Read the model definition and answer for the solid it produces. Units are mm, in the model's axes. A direction names the side the tool comes from. Round coordinates to 2 decimals unless told otherwise and drop trailing zeros. Write each loop counter-clockwise with the first axis right and the second up, starting at its lowest first coordinate (ties: lowest second). Pieces come first, ordered by that corner, then holes. Notation, with made-up numbers: (-1.75, 77.25) -> (43.25, 77.25) arc R4 ccw to (43.25, 82.25) -> close; hole circle Ø3 at (-38, 18). An arc over 180 degrees is marked (long way). Return JSON: item names as keys, results as strings.
from build123d import *

# Parameters (mm, degrees)
F0_R     = 6.3627
F1_DEPTH = 8.9916
F2_R     = 5.08
F3_DEPTH = 33.02
F4_DEPTH = 33.02


with BuildPart() as f1:
    # F0 (on Top) → F1 (new body)
    with BuildSketch(Plane.XY):
        Circle(F0_R)
    extrude(amount=-F1_DEPTH)

    # F2 (on Right) → F3 (join)
    with BuildSketch(Plane.YZ):
        with Locations((0, -3.8867404219)):
            Circle(F2_R)
    extrude(amount=F3_DEPTH)

    # F4 (cut, through all): a face of the model
    f4_faces = [f1.faces().sort_by_distance(p)[0] for p in [
        (0, 0, 0.4824606672),
    ]]
    extrude(f4_faces, amount=-F4_DEPTH, mode=Mode.SUBTRACT)


solid = f1.part
Item 1: Flat-ended cylindrical pins translate along their axes: pin 1 (1.5 mm diameter, centred on x = 6.5, y = 3.5, fed in from +Z); pin 2 (3 mm diameter, centred on x = 15, y = -4.5, fed in from -Z). Find the tip coordinate at first contact, or state that the pin passes through.
Worked answers:
{"pin 1": "stops at z = 0", "pin 2": "stops at z = -7.99"}
Item 2: Straight lines are drawn through the part: L1, parallel to Z at x = 19, y = -0.25; L2, parallel to Y at x = 29, z = -3.5; L3, parallel to Y at x = 8, z = -0.5. For each, find the intervals that lie inside material, in ascending order. Write a range as [from, to].
Worked answers:
{"L1": "z = [-8.96, 0]", "L2": "y = [-5.07, 5.07]", "L3": "y = [-3.79, 3.79]"}
Item 3: Section D-D (y = 2.5) is taken. Give the vertices of the cut face in (x, z), then the cut area to 3 significant figures.
Worked answers:
{"outline": "(-5.85, -8.99) -> (5.85, -8.99) -> (5.85, -8.31) -> (33.02, -8.31) -> (33.02, 0) -> (-5.85, 0) -> close", "area": "331 mm2"}
Item 4: A tool of negligible diameter and unlimited length cuts with its end or side. For faces 1 (the flat face through (13, 0, 0)), 2 (the cylindrical face through (18.221, -0.174, -8.964)), from which of +Z, -Z, +X, -X, +Y, -Y can it reach the whole face along a straight path? Write none if from no direction.
Worked answers:
{"face 1": "+Z, +X, -X, +Y, -Y", "face 2": "+X"}
Item 5: Section B-B (z = -3) is taken. Give the vertices of the cut face in (x, y), then the cut area to 3 significant figures.
Worked answers:
{"outline": "(3.93, -5) -> (33.02, -5) -> (33.02, 5) -> (3.93, 5) arc R6.36 ccw (long way) to start", "area": "401 mm2"}
Item 6: Section C-C (x = 11) is taken. Give the vertices of the cut face in (y, z), then the cut area to 3 significant figures.
Worked answers:
{"outline": "(-3.27, 0) arc R5.08 ccw (long way) to (3.27, 0) -> close", "area": "75.7 mm2"}
Item 7: Section A-A (y = 4.5) is taken. Give the vertices of the cut face in (x, z).
Worked answers:
{"outline": "(-4.5, -8.99) -> (4.5, -8.99) -> (4.5, -6.24) -> (33.02, -6.24) -> (33.02, -1.53) -> (4.5, -1.53) -> (4.5, 0) -> (-4.5, 0) -> close"}
